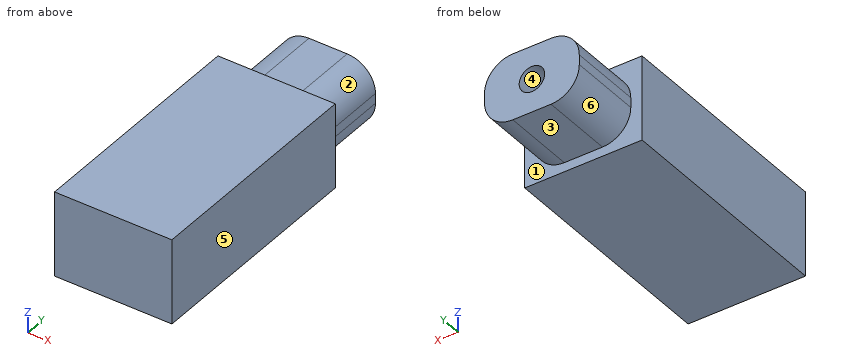
```python
from build123d import *

# Parameters (mm, degrees)
SKETCH1_W           = 21.082
SKETCH1_H           = 41.91
BOSS_EXTRUDE1_DEPTH = 15.24
BOSS_EXTRUDE2_DEPTH = 13.208
SKETCH3_R           = 2.286
CUT_EXTRUDE1_DEPTH  = 10.16


with BuildPart() as part:
    # Sketch1 → Boss-Extrude1 (new body)
    with BuildSketch(Plane.XY):
        Rectangle(SKETCH1_W, SKETCH1_H)
    extrude(amount=BOSS_EXTRUDE1_DEPTH)

    # Sketch2 → Boss-Extrude2 (add)
    with BuildSketch(Plane(origin=(0, 20.955, 0), x_dir=(1, 0, 0), z_dir=(0, 1, 0))):
        with BuildLine():
            Line((3.429, -13.589), (-3.429, -13.589))
            ThreePointArc((-3.429, -13.589), (-7.021102448, -12.101102448), (-8.509, -8.509))
            Line((-8.509, -8.509), (-8.509, -6.731))
            ThreePointArc((-8.509, -6.731), (-7.021102448, -3.138897552), (-3.429, -1.651))
            Line((-3.429, -1.651), (3.429, -1.651))
            ThreePointArc((3.429, -1.651), (7.021102448, -3.138897552), (8.509, -6.731))
            Line((8.509, -6.731), (8.509, -8.509))
            ThreePointArc((8.509, -8.509), (7.021102448, -12.101102448), (3.429, -13.589))
        make_face()
    extrude(amount=BOSS_EXTRUDE2_DEPTH)

    # Sketch3 → Cut-Extrude1 (cut)
    with BuildSketch(Plane(origin=(0, 34.163, 0), x_dir=(1, 0, 0), z_dir=(0, 1, 0))):
        with Locations(Location((0, -7.62, 0), (0, 0, 270))):
            Circle(SKETCH3_R)
    extrude(amount=-CUT_EXTRUDE1_DEPTH, mode=Mode.SUBTRACT)


solid = part.part
```
For this review, take the finished solid that the model builds, in its own axes (mm). Face numbers are marked on the shaded views. A direction names the side the tool comes from. Coordinates: 2 decimals unless noted, no trailing zeros. Write each loop counter-clockwise with the first axis right and the second up, starting at its lowest first coordinate (ties: lowest second). Pieces come first, ordered by that corner, then holes.
(1) Add section B-B on x = 0. Give the boundary of the cut face in (y, z) (3 decimals), then the cut area to 3 significant figures.
(2) The part is to be moulded in two halves that separate along X. For the marked faces 4, 5 and 6, say which applies: +X half, -X half, draft (parallel to the pull), parting line (faces both ways), or undercut.
(3) Wall thickness on probe 1 along X at (y, z) = (29.75, 7.62); probe 2 along Z at (x, y) = (-2.5, 25.5); probe 3 along Y at (x, z) = (-7, 2.25) (3 decimals): over which ranges is each line inside the solid? List them lowest first.
(4) For pin 1 Ø1.4 at (y, z) = (30.5, 7.5) entering from -X; pin 2 Ø2.5 at (x, z) = (-1, 8.5) entering from +Y; pin 3 Ø3.5 at (x, y) = (-1, 28.5) entering from -Z; pin 4 Ø4 at (x, z) = (0, 7.62) entering from +Y, all flat-tipped, find the tip position at first contact; note any pin that passes through.
(5) Add section A-A on y = 31. Give the boundary of the cut face in (x, z), then the cut area to 3 significant figures.
(6) Tool access review of the marked faces 1, 2 and 3: name each direction out of +Z, -Z, +X, -X, +Y, -Y from which nothing blocks a thin tool from reaching the whole face with its end or side.
(7) Add section D-D on x = 5.5. Give the boundary of the cut face in (y, z) (3 decimals).
(8) Add section C-C on z = 3.5. Give the boundary of the cut face in (x, y) (3 decimals), then the cut area to 3 significant figures.
Answer sheet:
1. outline: (-20.955, 0) - (20.955, 0) - (20.955, 1.651) - (34.163, 1.651) - (34.163, 5.334) - (24.003, 5.334) - (24.003, 9.906) - (34.163, 9.906) - (34.163, 13.589) - (20.955, 13.589) - (20.955, 15.24) - (-20.955, 15.24) - close
1. area: 750 mm2
2. face 4: undercut
2. face 5: +X half
2. face 6: -X half
3. probe 1: x = -8.51 to -2.29, 2.29 to 8.51
3. probe 2: z = 1.65 to 13.59
3. probe 3: y = -20.955 to 20.955
4. pin 1: stops at x = -8.51
4. pin 2: stops at y = 34.16
4. pin 3: stops at z = 1.65
4. pin 4: stops at y = 24
5. outline: (-8.51, 6.73) arc R5.08 ccw to (-3.43, 1.65) - (3.43, 1.65) arc R5.08 ccw to (8.51, 6.73) - (8.51, 8.51) arc R5.08 ccw to (3.43, 13.59) - (-3.43, 13.59) arc R5.08 ccw to (-8.51, 8.51) - close; hole circle Ø4.57 at (0, 7.62)
5. area: 165 mm2
6. face 1: +Y
6. face 2: +Z, +X, +Y
6. face 3: -Z, +X, -X, +Y
7. outline: (-20.955, 0) - (20.955, 0) - (20.955, 2.092) - (34.163, 2.092) - (34.163, 13.148) - (20.955, 13.148) - (20.955, 15.24) - (-20.955, 15.24) - close
8. outline: (-10.541, -20.955) - (10.541, -20.955) - (10.541, 20.955) - (7.349, 20.955) - (7.349, 34.163) - (-7.349, 34.163) - (-7.349, 20.955) - (-10.541, 20.955) - close
8. area: 1,080 mm2
